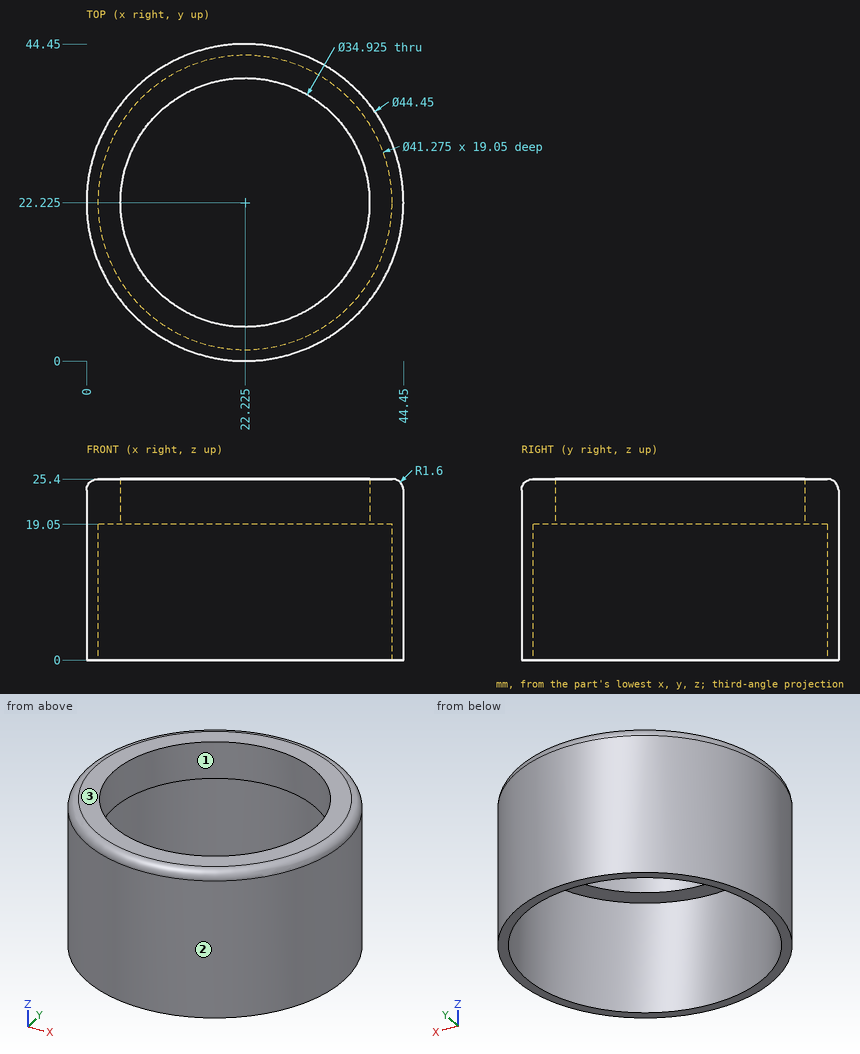
Design review of the part shown in the three views and the two pictorial views. Dimensions are in mm from the part's minimum x, y and z. Give positions to 0.01 mm unless a question says otherwise; leave off trailing zeros. Answer as a JSON object with one key per item and string values. Group by question number.
Q1. Insertion check: P1, Ø10, axis at x = 21, y = 5.5, coming from the +Z side; P2, Ø4, axis at y = 27, z = 4, coming from the +X side; P3, Ø8, axis at x = 30.5, z = 14.5, coming from the +Y side (3 decimals); P4, Ø6, axis at x = 27, z = 14.5, coming from the +Y side. Each pin has a flat end and moves straight along its axis. Give the tip position at first contact, or say it passes through.
Q2. For probe 1 along X at (y, z) = (6, 16.75) (1 decimal); probe 2 along Y at (x, z) = (14, 6.5); probe 3 along Y at (x, z) = (27, 15.25), list the stretches that pass through material, from the lowest coordinate up. Write a range as [from, to].
Q3. Mouldability with a two-part tool opening along Y and no side actions: class the marked faces 1, 2 and 3 as +Y half, -Y half, draft (parallel to the pull), parting line (faces both ways), or undercut.
Checked values:
{
 "1": {"P1": "z = 25.4", "P2": "x = 44.28", "P3": "y = 44.035", "P4": "y = 44.38"},
 "2": {"probe 1": "[7, 9.5], [35, 37.4]", "probe 2": "[1.58, 3.3], [41.15, 42.87]", "probe 3": "[0.52, 2.15], [42.3, 43.93]"},
 "3": {"face 1": "undercut", "face 2": "parting line", "face 3": "draft"}
}
